```python
from build123d import *

# Parameters (mm, degrees)
BOSS_EXTRUDE1_DEPTH = 0.8
SKETCH2_R           = 1.025
CUT_EXTRUDE2_DEPTH  = 10


# Read off the part's stored shape, not the designer's step: Boss-Extrude1
with BuildPart() as part:
    # Boss-Extrude1 outline → Boss-Extrude1 (new body)
    with BuildSketch(Plane.XY):
        with BuildLine():
            ThreePointArc((-2.3, 17.630609746), (-6.804111427, 16.426578088), (-10.840378111, 14.093069304))
            Line((-10.840378111, 14.093069304), (-25.865044656, 27.279258218))
            Line((-25.865044656, 27.279258218), (-27.279258218, 25.865044656))
            Line((-27.279258218, 25.865044656), (-14.093069304, 10.840378111))
            ThreePointArc((-14.093069304, 10.840378111), (-16.426578088, 6.804111427), (-17.630609746, 2.3))
            Line((-17.630609746, 2.3), (-37.578696944, 1))
            Line((-37.578696944, 1), (-37.578696944, -1))
            Line((-37.578696944, -1), (-17.630609746, -2.3))
            ThreePointArc((-17.630609746, -2.3), (-16.426578088, -6.804111427), (-14.093069304, -10.840378111))
            Line((-14.093069304, -10.840378111), (-27.279258218, -25.865044656))
            Line((-27.279258218, -25.865044656), (-25.865044656, -27.279258218))
            Line((-25.865044656, -27.279258218), (-10.840378111, -14.093069304))
            ThreePointArc((-10.840378111, -14.093069304), (-6.804111427, -16.426578088), (-2.3, -17.630609746))
            Line((-2.3, -17.630609746), (-1, -37.578696944))
            Line((-1, -37.578696944), (1, -37.578696944))
            Line((1, -37.578696944), (2.3, -17.630609746))
            ThreePointArc((2.3, -17.630609746), (6.804111427, -16.426578088), (10.840378111, -14.093069304))
            Line((10.840378111, -14.093069304), (25.865044656, -27.279258218))
            Line((25.865044656, -27.279258218), (27.279258218, -25.865044656))
            Line((27.279258218, -25.865044656), (14.093069304, -10.840378111))
            ThreePointArc((14.093069304, -10.840378111), (16.426578088, -6.804111427), (17.630609746, -2.3))
            Line((17.630609746, -2.3), (37.578696944, -1))
            Line((37.578696944, -1), (37.578696944, 1))
            Line((37.578696944, 1), (17.630609746, 2.3))
            ThreePointArc((17.630609746, 2.3), (16.426578088, 6.804111427), (14.093069304, 10.840378111))
            Line((14.093069304, 10.840378111), (27.279258218, 25.865044656))
            Line((27.279258218, 25.865044656), (25.865044656, 27.279258218))
            Line((25.865044656, 27.279258218), (10.840378111, 14.093069304))
            ThreePointArc((10.840378111, 14.093069304), (6.804111427, 16.426578088), (2.3, 17.630609746))
            Line((2.3, 17.630609746), (1, 37.578696944))
            Line((1, 37.578696944), (-1, 37.578696944))
            Line((-1, 37.578696944), (-2.3, 17.630609746))
        make_face()
        with BuildLine():
            Line((-1.5, -7), (-1.5, -4.769696007))
            ThreePointArc((-1.5, -4.769696007), (-5, 0), (-1.5, 4.769696007))
            Line((-1.5, 4.769696007), (-1.5, 7))
            Line((-1.5, 7), (1.5, 7))
            Line((1.5, 7), (1.5, 4.769696007))
            ThreePointArc((1.5, 4.769696007), (5, 0), (1.5, -4.769696007))
            Line((1.5, -4.769696007), (1.5, -7))
            Line((1.5, -7), (-1.5, -7))
        make_face(mode=Mode.SUBTRACT)
    extrude(amount=BOSS_EXTRUDE1_DEPTH)

    # Sketch2 → Cut-Extrude2 (cut)
    with BuildSketch(Plane.XY):
        with Locations((0, 20)):
            Circle(SKETCH2_R)
        with Locations((14.142135624, 14.142135624)):
            Circle(SKETCH2_R)
        with Locations((20, 0)):
            Circle(SKETCH2_R)
        with Locations((14.142135624, -14.142135624)):
            Circle(SKETCH2_R)
        with Locations((0, -20)):
            Circle(SKETCH2_R)
        with Locations((-14.142135624, -14.142135624)):
            Circle(SKETCH2_R)
        with Locations((-20, 0)):
            Circle(SKETCH2_R)
        with Locations((-14.142135624, 14.142135624)):
            Circle(SKETCH2_R)
    extrude(amount=CUT_EXTRUDE2_DEPTH, mode=Mode.SUBTRACT)


solid = part.part
```
Geometry check sheet. Reference: the model listing, model coordinates, mm. A direction names the side the tool comes from. Coordinates: 2 decimals unless noted, no trailing zeros. Order: outer loops, then holes, each group sorted by start corner. A loop starts at its lowest first (then second) coordinate and runs counter-clockwise, first axis right, second up. Notation, with made-up numbers: (41, 64) - (75, 64) arc R21 ccw to (75, 85) - close; hole circle Ø1 at (89, 51.5). An arc over 180 degrees is marked (long way). Answer as a JSON object with one key per item and string values. Group by question number.
Item 1: Scan lines: probe 1 along Y at (x, z) = (0, 0.1) (3 decimals); probe 2 along X at (y, z) = (0, 0.35) (3 decimals); probe 3 along X at (y, z) = (15.5, 0.35). Record each from-to range of solid material in increasing order.
Item 2: Draft check along X on faces 4 (the face through (-16.452, -6.744, 0.394)), 5 (the face through (5, 0.1, 0.4)), 6 (the face through (20.594, 18.248, 0.394)). Enter one of: +X half, -X half, draft (parallel to the pull), parting line (faces both ways), or undercut.
Item 3: Sectioned sample at A-A, the plane x = 0. Record the cut outline in (y, z) (3 decimals).
Item 4: Sectioned sample at C-C, the plane x = -23.5. Record the cut outline in (y, z), and give its area (3 significant figures).
Item 5: Depth check by flat-ended pin: pin 1 Ø1.5 at (x, y) = (24.5, 3) entering from +Z. Enter the tip coordinate at first touch or a pass-through.
Item 6: Tool access check on faces 1 (the face through (18.248, -20.594, 0.394)), 2 (the face through (16.452, 6.744, 0.394)), 3 (the face through (6.865, 16.401, 0.394)). Record the directions out of +Z, -Z, +X, -X, +Y, -Y that give a thin tool (end or side, any length) a straight path to the whole face; none if there is none.
Item 7: Sectioned sample at D-D, the plane z = 0.55. Give the number of separate pieces and of enclosed holes in the cut face, and give its area (3 significant figures).
Item 8: Sectioned sample at B-B, the plane y = -20. Record the cut outline in (x, z) (3 decimals), and give its area (3 significant figures).
Resolved:
{
 "1": {"probe 1": "-37.579 to -21.025, -18.975 to -7, 7 to 18.975, 21.025 to 37.579", "probe 2": "-37.579 to -21.025, -18.975 to -5, 5 to 18.975, 21.025 to 37.579", "probe 3": "-18.18 to -12.44, -8.71 to 8.71, 12.44 to 18.18"},
 "2": {"face 4": "-X half", "face 5": "undercut", "face 6": "+X half"},
 "3": {"outline": "(-37.579, 0) - (-21.025, 0) - (-21.025, 0.8) - (-37.579, 0.8) - close; (-18.975, 0) - (-7, 0) - (-7, 0.8) - (-18.975, 0.8) - close; (7, 0) - (18.975, 0) - (18.975, 0.8) - (7, 0.8) - close; (21.025, 0) - (37.579, 0) - (37.579, 0.8) - (21.025, 0.8) - close"},
 "4": {"outline": "(-25.2, 0) - (-21.56, 0) - (-21.56, 0.8) - (-25.2, 0.8) - close; (-1.92, 0) - (1.92, 0) - (1.92, 0.8) - (-1.92, 0.8) - close; (21.56, 0) - (25.2, 0) - (25.2, 0.8) - (21.56, 0.8) - close", "area": "8.90 mm^2"},
 "5": {"pin 1": "through"},
 "6": {"face 1": "+Z, -Z, -Y", "face 2": "+Z, -Z, +X", "face 3": "+Z, -Z, +Y"},
 "7": {"separate pieces": "1", "enclosed holes": "9", "area": "1,400 mm^2"},
 "8": {"outline": "(-22.132, 0) - (-17.571, 0) - (-17.571, 0.8) - (-22.132, 0.8) - close; (-2.146, 0) - (-1.025, 0) - (-1.025, 0.8) - (-2.146, 0.8) - close; (1.025, 0) - (2.146, 0) - (2.146, 0.8) - (1.025, 0.8) - close; (17.571, 0) - (22.132, 0) - (22.132, 0.8) - (17.571, 0.8) - close", "area": "9.09 mm^2"}
}
